from build123d import *

# Parameters (mm, degrees)
BOSS_EXTRUDE1_DEPTH = 1.5
CHAMFER1_SIZE2      = 1.091910703
CHAMFER1_SIZE       = 3
CUT_EXTRUDE1_DEPTH  = 69.98434605
FILLET1_R           = 1


with BuildPart() as part:
    # Sketch1 → Boss-Extrude1 (new, symmetric)
    with BuildSketch(Plane.XY):
        Polygon((-45, 0), (45, 0), (35.5, 52.2), (-35.5, 52.2), align=None)
    extrude(amount=BOSS_EXTRUDE1_DEPTH, both=True)

    # Chamfer1
    chamfer1_edges = [part.edges().sort_by_distance(p)[0] for p in [
        (0, 0, -1.5),
    ]]
    chamfer1_side = [part.faces().sort_by_distance(p)[0] for p in [
        (0, 0, -1.478161786),
    ]]
    chamfer(chamfer1_edges, length=CHAMFER1_SIZE - 0.0001, length2=CHAMFER1_SIZE2 - 0.0001, reference=chamfer1_side[0])  # a hair under: the kernel refuses the full size

    # Sketch2 → Cut-Extrude1 (cut, through all)
    with BuildSketch(Plane.XY.offset(1.5)):
        Polygon((-11, 37.2), (-11, 52.2), (-31, 52.2), (-31, 37.2), (-23, 37.2), align=None)
        with BuildLine():
            ThreePointArc((-9.219544457, 31.2), (-5.244044241, 27.530460197), (0, 26.2))
            Line((0, 26.2), (0, 52.2))
            Line((0, 52.2), (-11, 52.2))
            Line((-11, 52.2), (-11, 37.2))
            ThreePointArc((-11, 37.2), (-10.545496409, 34.070702078), (-9.219544457, 31.2))
        make_face()
        with BuildLine():
            Line((0, 52.2), (0, 26.2))
            ThreePointArc((0, 26.2), (7.778174593, 29.421825407), (11, 37.2))
            Line((11, 37.2), (11, 52.2))
            Line((11, 52.2), (0, 52.2))
        make_face()
        with BuildLine():
            ThreePointArc((0, 25), (-10, 15), (0, 5))
            Line((0, 5), (0, 25))
        make_face()
        with BuildLine():
            Line((0, 25), (0, 5))
            ThreePointArc((0, 5), (7.071067812, 7.928932188), (10, 15))
            ThreePointArc((10, 15), (7.071067812, 22.071067812), (0, 25))
        make_face()
        with BuildLine():
            Line((-23, 31.2), (-9.219544457, 31.2))
            ThreePointArc((-9.219544457, 31.2), (-10.545496409, 34.070702078), (-11, 37.2))
            Line((-11, 37.2), (-23, 37.2))
            Line((-23, 37.2), (-23, 31.2))
        make_face()
    extrude(amount=-CUT_EXTRUDE1_DEPTH, mode=Mode.SUBTRACT)

    # Fillet1
    fillet1_edges = [part.edges().sort_by_distance(p)[0] for p in [
        (-9.219544457, 31.2, 0),
        (-23, 31.2, 0),
        (-23, 37.2, 0),
        (-31, 37.2, 0),
    ]]
    fillet(fillet1_edges, radius=FILLET1_R)


solid = part.part
Verification items for the finished model (mm, model axes). A direction names the side the tool comes from. Coordinates: 2 decimals unless noted, no trailing zeros. Order: outer loops, then holes, each group sorted by start corner. A loop starts at its lowest first (then second) coordinate and runs counter-clockwise, first axis right, second up.
Item 1: Section check A-A, the plane y = 13.5. Enter the section's corners in (x, z), then the cut area to 3 significant figures.
Filled in:
outline: (-42.54, -1.5) - (-9.89, -1.5) - (-9.89, 1.5) - (-42.54, 1.5) - close; (9.89, -1.5) - (42.54, -1.5) - (42.54, 1.5) - (9.89, 1.5) - close
area: 196 mm2
Item 2: Material ranges on L1, parallel to X at y = 7.5, z = 1.3; L2, parallel to X at y = 16, z = 0.95; L3, parallel to Y at x = -8.5, z = 1, recorded low to high.
Filled in:
L1: x = -43.64 to -6.61, 6.61 to 43.64
L2: x = -42.09 to -9.95, 9.95 to 42.09
L3: y = 0.18 to 9.73, 20.27 to 30.22
Item 3: Access from +Z, -Z, +X, -X, +Y, -Y to the whole of each face (thin tool, end or side, straight path). Record for faces 1 (the face through (-40.184, 26.465, 0.021)), 2 (the face through (-23, 34, 0)).
Filled in:
face 1: +Z, -Z, -X, +Y
face 2: +Z, -Z, +Y
Item 4: Section check B-B, the plane z = 0. Enter the section's corners in (x, y).
Filled in:
outline: (-44.9, 0.55) - (44.9, 0.55) - (35.5, 52.2) - (11, 52.2) - (11, 37.2) arc R11 cw to (-8.93, 30.78) arc R1 ccw to (-9.75, 31.2) - (-22, 31.2) arc R1 cw to (-23, 32.2) - (-23, 36.2) arc R1 ccw to (-24, 37.2) - (-30, 37.2) arc R1 cw to (-31, 38.2) - (-31, 52.2) - (-35.5, 52.2) - close; hole circle Ø20 at (0, 15)
Item 5: Release check for a two-part mould opening along X. For faces 3 (the face through (9, 21, -1.5)), 4 (the face through (-16, 31.2, 0)), 5 (the face through (40.316, 25.735, 0.021)), 6 (the face through (-31, 45, 0)) record: +X half, -X half, draft (parallel to the pull), parting line (faces both ways), or undercut.
Filled in:
face 3: draft
face 4: undercut
face 5: +X half
face 6: undercut
